Could you check a few things on this model? Use its own coordinates, in mm. A direction names the side the tool comes from. Coordinates: 2 decimals unless noted, no trailing zeros. Write each loop counter-clockwise with the first axis right and the second up, starting at its lowest first coordinate (ties: lowest second). Pieces come first, ordered by that corner, then holes. Notation, with made-up numbers: M 69,89 L 112,89 A33 cw 112,124 Z; hole C 56,54 d11. An arc over 180 degrees is marked long. Write item = value, one per line.
```python
from build123d import *

# Parameters (mm, degrees)
F1_W     = 100
F1_H     = 100
F1_R     = 25
F2_DEPTH = 20
F3_W     = 15
F3_H     = 100
F4_DEPTH = 10


with BuildPart() as f2:
    # F1 (on face) → F2 (new body)
    with BuildSketch(Plane.XY):
        Rectangle(F1_W, F1_H)
        Circle(F1_R, mode=Mode.SUBTRACT)
    extrude(amount=F2_DEPTH)

    # F3 (on face) → F4 (cut)
    with BuildSketch(Plane.XY.offset(20)):
        with Locations((-37.5, 0)):
            Rectangle(F3_W, F3_H)
    extrude(amount=-F4_DEPTH, mode=Mode.SUBTRACT)


solid = f2.part
```
Item 1: Imagine slicing it at B-B (x = 0). Write out the boundary of the cut face in (y, z).
Numbers:
outline = M -50,0 L -25,0 L -25,20 L -50,20 Z; M 25,0 L 50,0 L 50,20 L 25,20 Z
Item 2: For faces 1 (the face through (27, 1, 20)), 2 (the face through (-45, -1, 15)), which set-ups out of +Z, -Z, +X, -X, +Y, -Y let a thin tool reach every point of the face, with its end or its side?
Numbers:
face_1 = +Z, +X, -X, +Y, -Y
face_2 = +Z, +Y, -Y
Item 3: If we mould it in two halves opening along X, with no side actions, what happens to faces 3 (the face through (-38, 1, 10)), 4 (the face through (-48, 1, 20)), 5 (the face through (50, -1, 10))? For each: pulls with the +X half, pulls with the -X half, needs draft (parallel to the pull), parting line crosses it, or undercut.
Numbers:
face_3 = undercut
face_4 = needs draft
face_5 = pulls with the +X half
Item 4: Imagine slicing it at C-C (y = 0). Write out the boundary of the cut face in (x, z).
Numbers:
outline = M -50,0 L -25,0 L -25,20 L -30,20 L -30,10 L -45,10 L -45,20 L -50,20 Z; M 25,0 L 50,0 L 50,20 L 25,20 Z
Item 5: If I drill on line 1 along Y through (x, z) = (0, 4.5); line 2 along X through (y, z) = (-9, 13.5); line 3 along X through (y, z) = (45, 14.25), over which ranges is the centre line in solid material (lowest first)?
Numbers:
line_1 = -50 to -25, 25 to 50
line_2 = -50 to -45, -30 to -23.32, 23.32 to 50
line_3 = -50 to -45, -30 to 50
Item 6: Imagine slicing it at A-A (z = 18.25). Write out the boundary of the cut face in (x, y).
Numbers:
outline = M -50,-50 L -45,-50 L -45,50 L -50,50 Z; M -30,-50 L 50,-50 L 50,50 L -30,50 Z; hole C 0,0 d50
Item 7: Imagine slicing it at D-D (z = 6.5). Write out the boundary of the cut face in (x, y).
Numbers:
outline = M -50,-50 L 50,-50 L 50,50 L -50,50 Z; hole C 0,0 d50
